Check sheet for the modelled part. Datum: model origin and axes. Units: mm. Face numbers are marked on the shaded views. A direction names the side the tool comes from. Round coordinates to 2 decimals unless told otherwise and drop trailing zeros. Order: outer loops, then holes, each group sorted by start corner. A loop starts at its lowest first (then second) coordinate and runs counter-clockwise, first axis right, second up.
Q1. Set-up check for the marked faces 4 and 5: record each of +Z, -Z, +X, -X, +Y, -Y from which the full face is reachable in a straight line by a thin tool's end or side.
Q2. Mould release check, pull along X, two halves, no side actions. Record for the marked faces 1, 2 and 3: +X half, -X half, draft (parallel to the pull), parting line (faces both ways), or undercut.
Q3. Depth check by flat-ended pin: P1, Ø12.5, axis at x = -79.5, y = 90, coming from the +Z side; P2, Ø4, axis at x = -79, z = 7, coming from the +Y side; P3, Ø3, axis at x = -92, z = 18, coming from the +Y side. Enter the tip coordinate at first touch or a pass-through.
Q4. Cross-section at B-B on x = -72. Record the cut outline in (y, z).
Q5. Scan lines: probe 1 along Y at (x, z) = (-139.5, 7); probe 2 along X at (y, z) = (107.5, 7); probe 3 along Y at (x, z) = (-78.5, 9.5). Record each from-to range of solid material in increasing order.
Q6. Cross-section at D-D on y = 91.5. Record the cut outline in (x, z), then the cut area to 3 significant figures.
Q7. Cross-section at C-C on z = 30. Record the cut outline in (x, y), then the cut area to 3 significant figures.
Q8. Cross-section at A-A on z = 9. Record the cut outline in (x, y), then the cut area to 3 significant figures.
Autodesk Inventor part; units mm, degrees
ref_plane "YZ Plane" through (0, 0, 0) normal (1, 0, 0) x (0, 1, 0)
ref_plane "XZ Plane" through (0, 0, 0) normal (0, 1, 0) x (-1, 0, 0)
ref_plane "XY Plane" through (0, 0, 0) normal (0, 0, 1) x (1, 0, 0)
sketch "Sketch1" plane through (0, 0, 0) normal (0, 0, 1) x (1, 0, 0)
  line L0 (0, 0) -> (-151, 0)
  line L1 (-151, 0) -> (-151, 112)
  line L2 (-151, 112) -> (0, 112)
  line L3 (0, 112) -> (0, 0)
  line L4 (-151, 0) -> (0, 0)
  line L5 (0, 0) -> (0, -1)
  line L6 (0, -1) -> (-151, -1)
  line L7 (-151, -1) -> (-151, 0)
  dimension "d0" = 151
  dimension "d1" = 112
  dimension "d35" = 1
extrude "Extrusion1" add sketch "Sketch1" along normal blind 3
sketch "Sketch2" plane through (0, 0, 3) normal (0, 0, 1) x (1, 0, 0)
  line L0 (-151, 0) -> (0, 0)
  line L1 (0, 0) -> (-151, 0)
  line L2 (-151, 0) -> (-151, 53)
  line L3 (-151, 53) -> (0, 53)
  line L4 (0, 53) -> (0, 0)
  line L5 (-148, 50) -> (-3, 50)
  line L6 (-3, 50) -> (-3, 3)
  line L7 (-3, 3) -> (-148, 3)
  line L8 (-148, 3) -> (-148, 50)
  line L9 (-151, -1) -> (0, -1)
  line L10 (-151, 112) -> (-151, -1)
  line L11 (0, -1) -> (0, 112)
  line L12 (-148, 3) -> (-3, 3)
  line L13 (-3, 3) -> (-3, 2)
  line L14 (-3, 2) -> (-148, 2)
  line L15 (-148, 2) -> (-148, 3)
  dimension "d4" = 151
  dimension "d5" = 53
  dimension "d6" = 3
  dimension "d7" = 3
  dimension "d8" = 3
  dimension "d9" = 3
  dimension "d36" = 1
extrude "Extrusion2" add sketch "Sketch2" along normal blind 30
sketch "Sketch3" plane through (0, 0, 3) normal (0, 0, 1) x (1, 0, 0)
  line L0 (-148, 109) -> (-103.5, 109)
  line L1 (-103.5, 109) -> (-103.5, 56)
  line L2 (-103.5, 56) -> (-148, 56)
  line L3 (-148, 56) -> (-148, 109)
  line L4 (-47.5, 109) -> (-3, 109)
  line L5 (-3, 109) -> (-3, 56)
  line L6 (-3, 56) -> (-47.5, 56)
  line L7 (-47.5, 56) -> (-47.5, 109)
  line L8 (0, 112) -> (-151, 112)
  line L9 (-151, 112) -> (-151, 53)
  line L10 (0, 53) -> (0, 112)
  line L11 (-85.5, 100) -> (-65.5, 100)
  line L12 (-65.5, 100) -> (-65.5, 65)
  line L13 (-65.5, 65) -> (-85.5, 65)
  line L14 (-85.5, 65) -> (-85.5, 100)
  line L15 (-62.5, 103) -> (-88.5, 103)
  line L16 (-88.5, 103) -> (-88.5, 62)
  line L17 (-88.5, 62) -> (-62.5, 62)
  line L18 (-62.5, 62) -> (-62.5, 103)
  line L19 (-100.5, 112) -> (-151, 112)
  line L20 (-151, 112) -> (-151, 53)
  line L21 (-151, 53) -> (-100.5, 53)
  line L22 (-100.5, 53) -> (-100.5, 112)
  line L23 (0, 112) -> (-50.5, 112)
  line L24 (-50.5, 112) -> (-50.5, 53)
  line L25 (-50.5, 53) -> (0, 53)
  line L26 (0, 53) -> (0, 112)
  point P0 (0, 0)
  dimension "d12" = 44.5
  dimension "d13" = 53
  dimension "d14" = 44.5
  dimension "d15" = 53
  dimension "d16" = 3
  dimension "d17" = 3
  dimension "d18" = 3
  dimension "d19" = 20
  dimension "d20" = 35
  dimension "d21" = 12
  dimension "d22" = 18
  dimension "d23" = 3
  dimension "d24" = 3
  dimension "d25" = 3
extrude "Extrusion3" add sketch "Sketch3" along normal blind 8
fillet "Fillet1" radius 4 6 edges at (-100.5, 82.5, 3) (-62.5, 82.5, 3) (-50.5, 82.5, 3) (-75.5, 103, 3) (-88.5, 82.5, 3) (-75.5, 62, 3)
sketch "Sketch6" plane through (-151, -1, 0) normal (0, -1, 0) x (1, 0, 0)
  line L0 (65.5, 21) -> (85.5, 21)
  line L1 (85.5, 21) -> (85.5, 18)
  line L2 (85.5, 18) -> (65.5, 18)
  line L3 (65.5, 18) -> (65.5, 21)
  line L4 (0, 0) -> (0, 33)
  line L5 (0, 33) -> (151, 33)
  point P0 (151, 0)
  dimension "d37" = 20
  dimension "d38" = 3
  dimension "d39" = 65.5
  dimension "d40" = 12
extrude "Extrusion5" cut sketch "Sketch6" against normal up to surface (54 mm away)
properties part number "bateria_mocowanie"
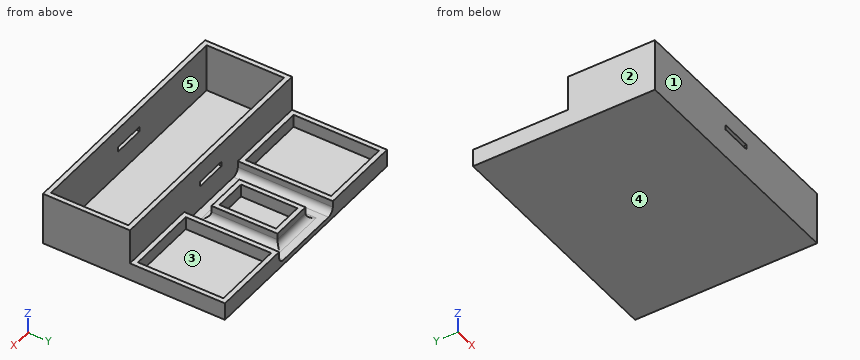
Results found:
1. face 4: -Z, +X, -X, +Y, -Y
1. face 5: +Z
2. face 1: draft
2. face 2: -X half
2. face 3: undercut
3. P1: stops at z = 11
3. P2: stops at y = 103.54
3. P3: stops at y = 53
4. outline: (-1, 0) - (112, 0) - (112, 3) - (107, 3) arc R4 cw to (103, 7) - (103, 11) - (100, 11) - (100, 3) - (65, 3) - (65, 11) - (62, 11) - (62, 7) arc R4 cw to (58, 3) - (53, 3) - (53, 18) - (50, 18) - (50, 3) - (2, 3) - (2, 18) - (-1, 18) - close; (-1, 21) - (2, 21) - (2, 33) - (-1, 33) - close; (50, 21) - (53, 21) - (53, 33) - (50, 33) - close
5. probe 1: y = -1 to 2, 50 to 56, 109 to 112
5. probe 2: x = -151 to -148, -103.5 to -100.5, -50.5 to -47.5, -3 to 0
5. probe 3: y = -1 to 2, 50 to 53, 62 to 65, 100 to 103
6. outline: (-151, 0) - (0, 0) - (0, 11) - (-3, 11) - (-3, 3) - (-47.5, 3) - (-47.5, 11) - (-50.5, 11) - (-50.5, 7) arc R4 cw to (-54.5, 3) - (-58.5, 3) arc R4 cw to (-62.5, 7) - (-62.5, 11) - (-65.5, 11) - (-65.5, 3) - (-85.5, 3) - (-85.5, 11) - (-88.5, 11) - (-88.5, 7) arc R4 cw to (-92.5, 3) - (-96.5, 3) arc R4 cw to (-100.5, 7) - (-100.5, 11) - (-103.5, 11) - (-103.5, 3) - (-148, 3) - (-148, 11) - (-151, 11) - close
6. area: 611 mm2
7. outline: (-151, -1) - (0, -1) - (0, 53) - (-151, 53) - close; hole (-148, 2) - (-3, 2) - (-3, 50) - (-148, 50) - close
7. area: 1,190 mm2
8. outline: (-151, -1) - (0, -1) - (0, 112) - (-50.5, 112) - (-50.5, 53) - (-100.5, 53) - (-100.5, 112) - (-151, 112) - close; (-88.5, 62) - (-62.5, 62) - (-62.5, 103) - (-88.5, 103) - close; hole (-148, 2) - (-3, 2) - (-3, 50) - (-148, 50) - close; hole (-148, 56) - (-103.5, 56) - (-103.5, 109) - (-148, 109) - close; hole (-85.5, 65) - (-65.5, 65) - (-65.5, 100) - (-85.5, 100) - close; hole (-47.5, 56) - (-3, 56) - (-3, 109) - (-47.5, 109) - close
8. area: 2,800 mm2
